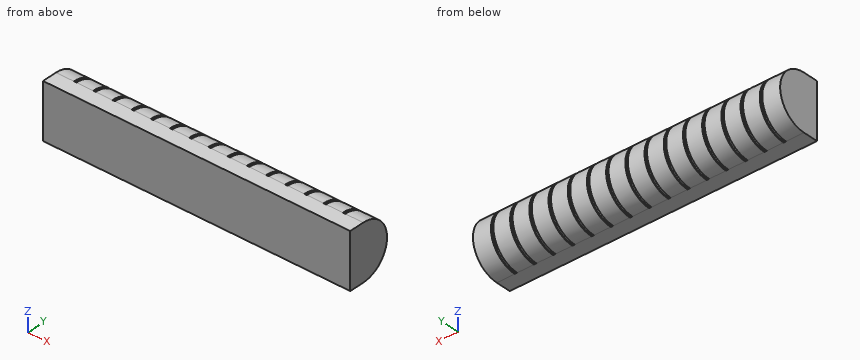
Autodesk Fusion 360 part; units mm, degrees
sketch "Sketch1" plane through (0, 0, 0) normal (1, 0, 0) x (0, 1, 0)
  circle A0 centre (0, 0) radius 2.75
  line L0 (0, 0) -> (0, 2.75) construction
  line L1 (0, 0) -> (0, -2.75) construction
  line L2 (0, 2.75) -> (-1.5, 2.75)
  line L3 (-1.5, 2.75) -> (-1.5, -2.75)
  line L4 (-1.5, -2.75) -> (0, -2.75)
  line L5 (0, -2.75) -> (0, 2.75)
  dimension "d1" = 5.5
  dimension "d79" = 1.5
extrude "Extrude1" add sketch "Sketch1" along normal mid plane 30.8 contours A0 L5 | A0 L3 L5 | A0 L3
ref_plane "WorkPlane1" through (0, 0, 0) normal (1, 0, 0) x (0, 1, 0)
sketch "Sketch2" plane through (0, 0, 0) normal (1, 0, 0) x (0, 1, 0)
  circle A0 centre (0, 0) radius 2.75
  circle A1 centre (0, 0) radius 2.625
  dimension "d5" = 5.5
  dimension "d6" = 5.25
extrude "Extrude2" cut sketch "Sketch2" along normal mid plane 0.25
ref_plane "WorkPlane2" through (7.7, 0, 0) normal (1, 0, 0) x (0, 1, 0)
sketch "Sketch3" plane through (7.7, 0, 0) normal (1, 0, 0) x (0, 1, 0)
  circle A0 centre (0, 0) radius 2.75
  circle A1 centre (0, 0) radius 2.625
  dimension "d10" = 5.5
  dimension "d11" = 5.25
extrude "Extrude3" cut sketch "Sketch3" along normal mid plane 0.25
ref_plane "WorkPlane3" through (11.55, 0, 0) normal (1, 0, 0) x (0, 1, 0)
sketch "Sketch4" plane through (11.55, 0, 0) normal (1, 0, 0) x (0, 1, 0)
  circle A0 centre (0, 0) radius 2.75
  circle A1 centre (0, 0) radius 2.625
  dimension "d15" = 5.5
  dimension "d16" = 5.25
extrude "Extrude4" cut sketch "Sketch4" along normal mid plane 0.25
ref_plane "WorkPlane4" through (13.475, 0, 0) normal (1, 0, 0) x (0, 1, 0)
sketch "Sketch5" plane through (13.475, 0, 0) normal (1, 0, 0) x (0, 1, 0)
  circle A0 centre (0, 0) radius 2.75
  circle A1 centre (0, 0) radius 2.625
  dimension "d20" = 5.5
  dimension "d21" = 5.25
extrude "Extrude5" cut sketch "Sketch5" along normal mid plane 0.25
ref_plane "WorkPlane5" through (9.625, 0, 0) normal (1, 0, 0) x (0, 1, 0)
sketch "Sketch6" plane through (9.625, 0, 0) normal (1, 0, 0) x (0, 1, 0)
  circle A0 centre (0, 0) radius 2.75
  circle A1 centre (0, 0) radius 2.625
  dimension "d25" = 5.5
  dimension "d26" = 5.25
extrude "Extrude6" cut sketch "Sketch6" along normal mid plane 0.25
ref_plane "WorkPlane6" through (5.775, 0, 0) normal (1, 0, 0) x (0, 1, 0)
sketch "Sketch7" plane through (5.775, 0, 0) normal (1, 0, 0) x (0, 1, 0)
  circle A0 centre (0, 0) radius 2.75
  circle A1 centre (0, 0) radius 2.625
  dimension "d30" = 5.5
  dimension "d31" = 5.25
extrude "Extrude7" cut sketch "Sketch7" along normal mid plane 0.25
ref_plane "WorkPlane7" through (3.85, 0, 0) normal (1, 0, 0) x (0, 1, 0)
sketch "Sketch8" plane through (3.85, 0, 0) normal (1, 0, 0) x (0, 1, 0)
  circle A0 centre (0, 0) radius 2.75
  circle A1 centre (0, 0) radius 2.625
  dimension "d35" = 5.5
  dimension "d36" = 5.25
extrude "Extrude8" cut sketch "Sketch8" along normal mid plane 0.25
ref_plane "WorkPlane8" through (1.925, 0, 0) normal (1, 0, 0) x (0, 1, 0)
sketch "Sketch9" plane through (1.925, 0, 0) normal (1, 0, 0) x (0, 1, 0)
  circle A0 centre (0, 0) radius 2.75
  circle A1 centre (0, 0) radius 2.625
  dimension "d40" = 5.5
  dimension "d41" = 5.25
extrude "Extrude9" cut sketch "Sketch9" along normal mid plane 0.25
ref_plane "WorkPlane9" through (-13.475, 0, 0) normal (-1, 0, 0) x (0, -1, 0)
sketch "Sketch10" plane through (-13.475, 0, 0) normal (-1, 0, 0) x (0, 1, 0)
  circle A0 centre (0, 0) radius 2.75
  circle A1 centre (0, 0) radius 2.625
  dimension "d45" = 5.5
  dimension "d46" = 5.25
extrude "Extrude10" cut sketch "Sketch10" along normal mid plane 0.25
ref_plane "WorkPlane10" through (-11.55, 0, 0) normal (-1, 0, 0) x (0, -1, 0)
sketch "Sketch11" plane through (-11.55, 0, 0) normal (-1, 0, 0) x (0, 1, 0)
  circle A0 centre (0, 0) radius 2.75
  circle A1 centre (0, 0) radius 2.625
  dimension "d50" = 5.5
  dimension "d51" = 5.25
extrude "Extrude11" cut sketch "Sketch11" along normal mid plane 0.25
ref_plane "WorkPlane11" through (-9.625, 0, 0) normal (-1, 0, 0) x (0, -1, 0)
sketch "Sketch12" plane through (-9.625, 0, 0) normal (-1, 0, 0) x (0, 1, 0)
  circle A0 centre (0, 0) radius 2.75
  circle A1 centre (0, 0) radius 2.625
  dimension "d55" = 5.5
  dimension "d56" = 5.25
extrude "Extrude12" cut sketch "Sketch12" along normal mid plane 0.25
ref_plane "WorkPlane12" through (-7.7, 0, 0) normal (-1, 0, 0) x (0, -1, 0)
sketch "Sketch13" plane through (-7.7, 0, 0) normal (-1, 0, 0) x (0, 1, 0)
  circle A0 centre (0, 0) radius 2.75
  circle A1 centre (0, 0) radius 2.625
  dimension "d60" = 5.5
  dimension "d61" = 5.25
extrude "Extrude13" cut sketch "Sketch13" along normal mid plane 0.25
ref_plane "WorkPlane13" through (-5.775, 0, 0) normal (-1, 0, 0) x (0, -1, 0)
sketch "Sketch14" plane through (-5.775, 0, 0) normal (-1, 0, 0) x (0, 1, 0)
  circle A0 centre (0, 0) radius 2.75
  circle A1 centre (0, 0) radius 2.625
  dimension "d65" = 5.5
  dimension "d66" = 5.25
extrude "Extrude14" cut sketch "Sketch14" along normal mid plane 0.25
ref_plane "WorkPlane14" through (-3.85, 0, 0) normal (-1, 0, 0) x (0, -1, 0)
sketch "Sketch15" plane through (-3.85, 0, 0) normal (-1, 0, 0) x (0, 1, 0)
  circle A0 centre (0, 0) radius 2.75
  circle A1 centre (0, 0) radius 2.625
  dimension "d70" = 5.5
  dimension "d71" = 5.25
extrude "Extrude15" cut sketch "Sketch15" along normal mid plane 0.25
ref_plane "WorkPlane15" through (-1.925, 0, 0) normal (-1, 0, 0) x (0, -1, 0)
sketch "Sketch16" plane through (-1.925, 0, 0) normal (-1, 0, 0) x (0, 1, 0)
  circle A0 centre (0, 0) radius 2.75
  circle A1 centre (0, 0) radius 2.625
  dimension "d75" = 5.5
  dimension "d76" = 5.25
extrude "Extrude16" cut sketch "Sketch16" along normal mid plane 0.25
extrude "Extrude17" add sketch "Sketch1" along normal mid plane 30.8 contours A0 L3 L5 | A0 L2 L3 | A0 L3 L4
extrude "Extrude18" cut sketch "Sketch1" along normal mid plane 30.8 contours A0 L3
Read the model definition and answer for the solid it produces. Units are mm, in the model's axes. Give positions to 0.01 mm unless a question says otherwise; leave off trailing zeros. Loops run counter-clockwise (first coordinate to the right, second up) from the corner with the lowest first, then second, coordinate; pieces in that order, holes last.
Item 1: Each of these flat-tipped pins is pushed along its axis until it touches: pin 1 Ø1.5 at (x, y) = (-5, 0.5) entering from +Z; pin 2 Ø1 at (x, y) = (-11.5, 2) entering from -Z; pin 3 Ø1.5 at (x, y) = (-4.5, 1) entering from +Z. Where does it stop, or does it pass through?
Item 2: Find the intervals of material crossed by line 1 along Y through (x, z) = (10, 1.5); line 2 along Z through (x, y) = (3, 0.5); line 3 along Y through (x, z) = (-0.5, -2.1), in increasing order.
Item 3: The part is cut by section A-A (x = -1.5). Write down the section's boundary in (y, z).
Taken from the geometry:
1. pin 1: stops at z = 2.75
1. pin 2: stops at z = -2.3
1. pin 3: stops at z = 2.74
2. line 1: y = -1.5 to 2.3
2. line 2: z = -2.7 to 2.7
2. line 3: y = -1.5 to 1.78
3. outline: (-1.5, -2.75) - (0, -2.75) arc R2.75 ccw to (0, 2.75) - (-1.5, 2.75) - close
